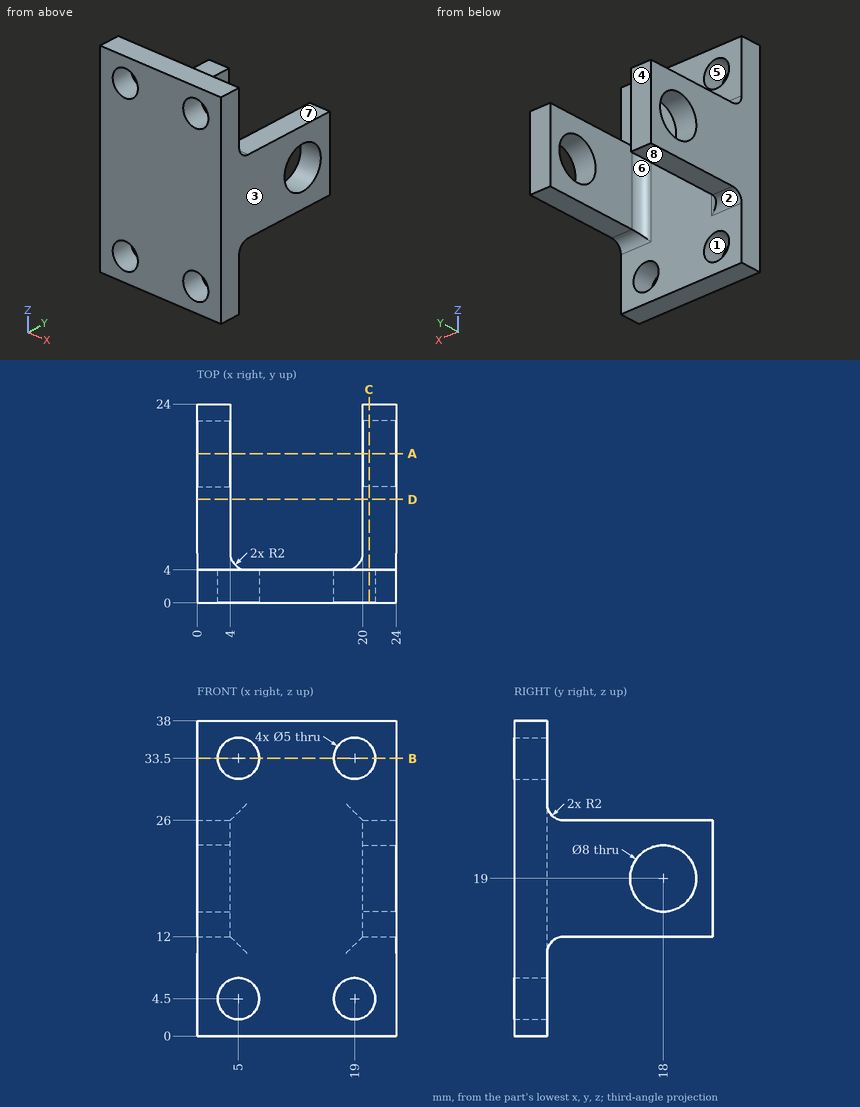
Could you check a few things on this drawing? It's one solid part, dimensions in mm from its lowest x, y, z. A direction names the side the tool comes from. Coordinates: 2 decimals unless noted, no trailing zeros. Order: outer loops, then holes, each group sorted by start corner. A loop starts at its lowest first (then second) coordinate and runs counter-clockwise, first axis right, second up. Notation, with made-up numbers: M -7.75,71.5 L 25.25,71.5 A12 ccw 25.25,81.5 Z; hole C 75,86.25 d8. An arc over 180 degrees is marked long. Answer as a JSON object with one key per item and string values. Group by question number.
(1) Suppose I cut it at C-C, the plane x = 20.75. Please give me the cut outline in (y, z), then the cut area to 3 significant figures.
(2) For pin 1 (4.5 mm diameter, centred on x = 21.5, y = 13, fed in from +Z); pin 2 (6 mm diameter, centred on x = 5, z = 4.5, fed in from +Y); pin 3 (4.5 mm diameter, centred on x = 1.5, y = 19, fed in from -Z), each with a flat end and sliding along its axis, tell me the tip position at first contact or that it passes through.
(3) Suppose I cut it at A-A, the plane y = 18. Please give me the cut outline in (x, z).
(4) Which directions (+Z, -Z, +X, -X, +Y, -Y) give clear straight access to the entire face, cutting with the end or side of a thin tool? Please do the marked faces 4, 5, 6, 7 and 8.
(5) If we mould it in two halves opening along Z, with no side actions, what happens to the marked faces 1, 2 and 3? For each: released by +Z, released by -Z, zero draft, split by the parting line, or undercut.
(6) I need wall thicknesses on probe 1 along X at (y, z) = (2.25, 4.5); probe 2 along Z at (x, y) = (19, 1.9); probe 3 along Y at (x, z) = (21.9, 19). Which ranges of each line are inside material? Lowest first, please.
(7) Suppose I cut it at B-B, the plane z = 33.5. Please give me the cut outline in (x, y).
(8) Suppose I cut it at D-D, the plane y = 12.5. Please give me the cut outline in (x, z), then the cut area to 3 significant figures.
Values found:
{
 "1": {"outline": "M 0,0 L 4,0 L 4,2.71 L 0,2.71 Z; M 0,6.29 L 4,6.29 L 4,10 A2 cw 6,12 L 24,12 L 24,26 L 6,26 A2 cw 4,28 L 4,31.71 L 0,31.71 Z; M 0,35.29 L 4,35.29 L 4,38 L 0,38 Z; hole C 18,19 d8", "area": "355 mm^2"},
 "2": {"pin 1": "stops at z = 26", "pin 2": "stops at y = 4", "pin 3": "stops at z = 12"},
 "3": {"outline": "M 0,12 L 4,12 L 4,15 L 0,15 Z; M 0,23 L 4,23 L 4,26 L 0,26 Z; M 20,12 L 24,12 L 24,15 L 20,15 Z; M 20,23 L 24,23 L 24,26 L 20,26 Z"},
 "4": {"face 4": "+Z, -Z, +X, -X, +Y", "face 5": "+Y, -Y", "face 6": "+Z, -Z, +Y", "face 7": "+Z, +X, -X, +Y", "face 8": "-Z, +X, -X, +Y"},
 "5": {"face 1": "undercut", "face 2": "released by -Z", "face 3": "zero draft"},
 "6": {"probe 1": "x = 0 to 2.5, 7.5 to 16.5, 21.5 to 24", "probe 2": "z = 0 to 2, 7 to 31, 36 to 38", "probe 3": "y = 0 to 14, 22 to 24"},
 "7": {"outline": "M 0,0 L 2.5,0 L 2.5,4 L 0,4 Z; M 7.5,0 L 16.5,0 L 16.5,4 L 7.5,4 Z; M 21.5,0 L 24,0 L 24,4 L 21.5,4 Z"},
 "8": {"outline": "M 0,12 L 4,12 L 4,26 L 0,26 Z; M 20,12 L 24,12 L 24,26 L 20,26 Z", "area": "112 mm^2"}
}
